```python
from build123d import *

# Parameters (mm, degrees)
SKETCH1_W           = 38
SKETCH1_H           = 81
BOSS_EXTRUDE1_DEPTH = 3
BOSS_EXTRUDE2_DEPTH = 7


with BuildPart() as part:
    # Sketch1 → Boss-Extrude1 (new body)
    with BuildSketch(Plane.XY):
        with Locations((0, -38)):
            Rectangle(SKETCH1_W, SKETCH1_H)
    extrude(amount=BOSS_EXTRUDE1_DEPTH)

    # Sketch2 → Boss-Extrude2 (add)
    with BuildSketch(Plane(origin=(0, 0, 0), x_dir=(-1, 0, 0), z_dir=(0, 0, -1))):
        Polygon((-19, -5.5), (-19, 2.5), (19, 2.5), (19, -5.5), (16.2, -5.5), (16.2, 1.2), (-16.2, 1.2), (-16.2, -5.5), align=None)
        Polygon((-16.2, -77.2), (16.2, -77.2), (16.2, -70.5), (19, -70.5), (19, -78.5), (-19, -78.5), (-19, -70.5), (-16.2, -70.5), align=None)
    extrude(amount=BOSS_EXTRUDE2_DEPTH)


solid = part.part
```
The listing builds one solid part. Answer for the finished solid, in the listing's coordinates (mm). A direction names the side the tool comes from. Give positions to 0.01 mm unless a question says otherwise; leave off trailing zeros. Write each loop counter-clockwise with the first axis right and the second up, starting at its lowest first coordinate (ties: lowest second). Pieces come first, ordered by that corner, then holes. Notation, with made-up numbers: (65, 2.25) -> (74, 2.25) arc R6 cw to (74, 8.25) -> close; hole circle Ø10 at (-28, -7.5). An arc over 180 degrees is marked (long way). Use one line per item in the form item = value.
1) Section A-A on z = -1.5 is taken. Write down the section's boundary in (x, y).
Result:
outline = (-19, -78.5) -> (19, -78.5) -> (19, -70.5) -> (16.2, -70.5) -> (16.2, -77.2) -> (-16.2, -77.2) -> (-16.2, -70.5) -> (-19, -70.5) -> close; (-19, -5.5) -> (-16.2, -5.5) -> (-16.2, 1.2) -> (16.2, 1.2) -> (16.2, -5.5) -> (19, -5.5) -> (19, 2.5) -> (-19, 2.5) -> close
2) For a pull along Y with two mould halves and no side action, classify faces 1 (the flat face through (0, -78, -7)), 2 (the flat face through (-18, -70.5, -3)), 3 (the flat face through (0, -78.5, -2)) as +Y half, -Y half, draft (parallel to the pull), parting line (faces both ways), or undercut.
Result:
face_1 = draft
face_2 = undercut
face_3 = -Y half
3) Section B-B on y = -73 is taken. Write down the section's boundary in (x, z), plus the area to 3 significant figures.
Result:
outline = (-19, -7) -> (-16.2, -7) -> (-16.2, 0) -> (16.2, 0) -> (16.2, -7) -> (19, -7) -> (19, 3) -> (-19, 3) -> close
area = 153 mm²
4) A tool of negligible diameter and unlimited length cuts with its end or side. For faces 4 (the flat face through (18, -5.5, -3)), 5 (the flat face through (0, 2.5, -2)), 6 (the flat face through (16.2, -2, -3)), from which of +Z, -Z, +X, -X, +Y, -Y can it reach the whole face along a straight path? Write none if from no direction.
Result:
face_4 = -Z, +X, -X
face_5 = +Z, -Z, +X, -X, +Y
face_6 = -Z
5) Straight lines are drawn through the part: probe 1 along Y at (x, z) = (-8, -1); probe 2 along Y at (x, z) = (17, -5.25); probe 3 along Z at (x, y) = (2.5, -52.5). For each, find the intervals that lie inside material, in ascending order.
Result:
probe_1 = -78.5 to -77.2, 1.2 to 2.5
probe_2 = -78.5 to -70.5, -5.5 to 2.5
probe_3 = 0 to 3
6) This flat-tipped pin is pushed along its axis until it touches: P1, Ø12, axis at x = 12, y = -49, coming from the -Z side. Where does it stop, or does it pass through?
Result:
P1 = 0
7) Section C-C on x = -8.5 is taken. Write down the section's boundary in (y, z), plus the area to 3 significant figures.
Result:
outline = (-78.5, -7) -> (-77.2, -7) -> (-77.2, 0) -> (1.2, 0) -> (1.2, -7) -> (2.5, -7) -> (2.5, 3) -> (-78.5, 3) -> close
area = 261 mm²
8) Section D-D on y = -62 is taken. Write down the section's boundary in (x, z), plus the area to 3 significant figures.
Result:
outline = (-19, 0) -> (19, 0) -> (19, 3) -> (-19, 3) -> close
area = 114 mm²
